```python
from build123d import *

# Parameters (mm, degrees)
PAD_DEPTH    = 1
PAD001_DEPTH = 0.5


with BuildPart() as part:
    # Sketch → Pad (new body)
    with BuildSketch(Plane.XY):
        with BuildLine():
            Line((-3, -16), (3, -16))
            Line((3, -16), (3, 3.534144))
            ThreePointArc((3, 3.534144), (-0.096514, 3.144536), (-3, 2))
            Line((-3, -16), (-3, 2))
        make_face()
    extrude(amount=PAD_DEPTH)

    # Sketch001 → Pad001 (new body)
    with BuildSketch(Plane.XY.offset(1)):
        Polygon((-2.5, 1.5), (2.5, 1.5), (2.5, 0.5), (-1.5, -6.5), (2.5, -6.5), (2.5, -7.5), (-1.5, -14.5), (2.5, -14.5), (2.5, -15.5), (-2.5, -15.5), (-2.5, -14.5), (1.621962, -7.5), (-2.378038, -7.5), (-2.378038, -6.5), (1.5, 0.5), (-2.5, 0.5), align=None)
    extrude(amount=PAD001_DEPTH)


solid = part.part
```
Model file for the job. Use its own axes, mm. A direction names the side the tool comes from. Give positions to 0.01 mm unless a question says otherwise; leave off trailing zeros. Loops run counter-clockwise (first coordinate to the right, second up) from the corner with the lowest first, then second, coordinate; pieces in that order, holes last. Notation, with made-up numbers: (-13, 32) -> (25, 32) arc R16 cw to (25, 36) -> close; hole circle Ø4 at (-24.5, -16). An arc over 180 degrees is marked (long way). Write each question's results on one line, items separated by ' | '.
(1) Flat gauge pins, fed straight in: pin 1 Ø3 at (x, y) = (-0.5, -14) entering from +Z; pin 2 Ø0.6 at (y, z) = (-7, 1.5) entering from +X. Where does each tip first touch, or does it go through?
Geometry results:
pin 1: stops at z = 1.5 | pin 2: stops at x = 2.5
(2) Probe line 1 along Y through (x, z) = (-1, 1.1) (3 decimals); line 2 along Y through (x, z) = (0.5, 1.25); line 3 along Y through (x, z) = (2.25, 1.15). List the from-to ranges inside material, lowest first.
Geometry results:
line 1: y = -15.5 to -14.5, -13.625 to -11.953, -7.5 to -6.5, -5.625 to -4.013, 0.5 to 1.5 | line 2: y = -15.5 to -14.5, -11 to -9.41, -7.5 to -6.5, -3 to -1.31, 0.5 to 1.5 | line 3: y = -15.5 to -14.5, -7.94 to -6.5, 0.06 to 1.5
(3) Tool access for faces 1 (the flat face through (-0.466, -3.049, 1.246)), 2 (the flat face through (0, -16, 0.5)), 3 (the flat face through (0.5, -3, 1.2)): list every direction of +Z, -Z, +X, -X, +Y, -Y with a clear straight run to the whole face (end or side of a thin tool).
Geometry results:
face 1: +Z, -X | face 2: +Z, -Z, +X, -X, -Y | face 3: +Z, +X
(4) Cut at C-C on y = -14.25. List the corners of the cut face in (x, z), and give its area (3 significant figures).
Geometry results:
outline: (-3, 0) -> (3, 0) -> (3, 1) -> (-1.36, 1) -> (-1.36, 1.5) -> (-2.35, 1.5) -> (-2.35, 1) -> (-3, 1) -> close | area: 6.50 mm²
(5) Cut at A-A on z = 1.2. List the corners of the cut face in (x, y), and give its area (3 significant figures).
Geometry results:
outline: (-2.5, -15.5) -> (2.5, -15.5) -> (2.5, -14.5) -> (-1.5, -14.5) -> (2.5, -7.5) -> (2.5, -6.5) -> (-1.5, -6.5) -> (2.5, 0.5) -> (2.5, 1.5) -> (-2.5, 1.5) -> (-2.5, 0.5) -> (1.5, 0.5) -> (-2.38, -6.5) -> (-2.38, -7.5) -> (1.62, -7.5) -> (-2.5, -14.5) -> close | area: 28.0 mm²
(6) Cut at B-B on x = 1.25. List the corners of the cut face in (y, z), and give its area (3 significant figures).
Geometry results:
outline: (-16, 0) -> (3.41, 0) -> (3.41, 1) -> (1.5, 1) -> (1.5, 1.5) -> (0.5, 1.5) -> (0.5, 1) -> (0.05, 1) -> (0.05, 1.5) -> (-1.69, 1.5) -> (-1.69, 1) -> (-6.5, 1) -> (-6.5, 1.5) -> (-7.5, 1.5) -> (-7.5, 1) -> (-8.13, 1) -> (-8.13, 1.5) -> (-9.69, 1.5) -> (-9.69, 1) -> (-14.5, 1) -> (-14.5, 1.5) -> (-15.5, 1.5) -> (-15.5, 1) -> (-16, 1) -> close | area: 22.6 mm²
(7) Cut at D-D on x = -1.75. List the corners of the cut face in (y, z).
Geometry results:
outline: (-16, 0) -> (2.6, 0) -> (2.6, 1) -> (1.5, 1) -> (1.5, 1.5) -> (0.5, 1.5) -> (0.5, 1) -> (-5.37, 1) -> (-5.37, 1.5) -> (-7.5, 1.5) -> (-7.5, 1) -> (-13.23, 1) -> (-13.23, 1.5) -> (-15.5, 1.5) -> (-15.5, 1) -> (-16, 1) -> close
(8) Pull direction Y, two halves, no side cores. Call faces 4 (the flat face through (0, -6, 0)), 5 (the flat face through (-0.47, -11.05, 1.25)), 6 (the cylindrical face through (-0.054, 3.155, 0.493)): released by +Y, released by -Y, zero draft, split by the parting line, or undercut.
Geometry results:
face 4: zero draft | face 5: undercut | face 6: released by +Y
